Autodesk Inventor part; units mm, degrees
ref_plane "YZ Plane" through (0, 0, 0) normal (1, 0, 0) x (0, 1, 0)
ref_plane "XZ Plane" through (0, 0, 0) normal (0, 1, 0) x (-1, 0, 0)
ref_plane "XY Plane" through (0, 0, 0) normal (0, 0, 1) x (1, 0, 0)
sketch "Sketch1" plane through (0, 0, 0) normal (0, 0, 1) x (1, 0, 0)
  line L0 (0, 0) -> (76.2, 0)
  line L1 (0, 0) -> (0, -50.8)
  line L2 (0, -50.8) -> (12.7, -50.8)
  line L3 (18.3796, -49.4592) -> (69.1796, -24.0592)
  arc A0 (12.7, -50.8) -> (18.3796, -49.4592) centre (12.7, -38.1) ccw
  line L4 (76.2, 0) -> (76.2, -12.7)
  arc A1 (69.1796, -24.0592) -> (76.2, -12.7) centre (63.5, -12.7) ccw
  circle A2 centre (12.7, -38.1) radius 4.8006
  circle A3 centre (12.7, -12.7) radius 4.8006
  circle A4 centre (63.5, -12.7) radius 4.8006
  line L5 (12.7, -12.7) -> (63.5, -12.7) construction
  line L6 (12.7, -38.1) -> (12.7, -12.7) construction
  circle A5 centre (38.1, -25.4) radius 3.175
  dimension "d2" = 50.8
  dimension "d3" = 12.7
  dimension "d4" = 12.7
  dimension "d5" = 12.7
  dimension "d7" = 9.6012
  dimension "d8" = 25.4
  dimension "d10" = 50.8
  dimension "d11" = 12.7
  dimension "d12" = 6.35
  dimension "d13" = 12.7
  dimension "d14" = 25.4
  dimension "d15" = 12.7
  dimension "d16" = 76.2
extrude "Extrusion1" add sketch "Sketch1" along normal mid plane 9.525
properties part number "Plate"
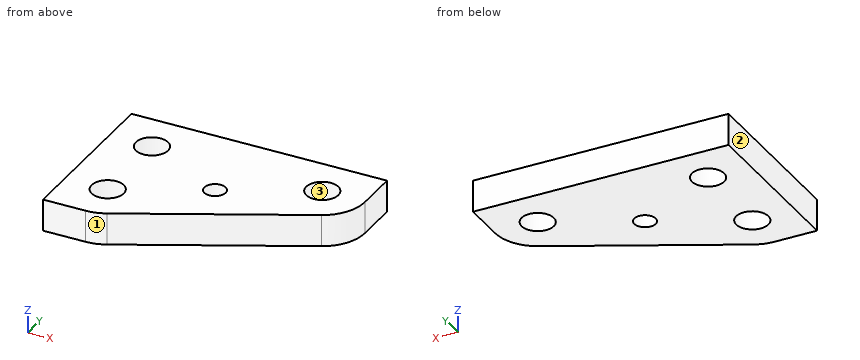
Verification items for the finished model (mm, model axes). Face numbers are marked on the shaded views. Round coordinates to 2 decimals unless told otherwise and drop trailing zeros. Loops run counter-clockwise (first coordinate to the right, second up) from the corner with the lowest first, then second, coordinate; pieces in that order, holes last. Notation, with made-up numbers: (64, 79.25) - (71, 79.25) arc R28 ccw to (71, 115.25) - close; hole circle Ø8 at (68.25, 61.5). An arc over 180 degrees is marked (long way). Answer in a Markdown table with one row per item. Add a question column.
Q1. Section check D-D on x = 15. Enter the section's corners in (y, z), plus the area to 3 significant figures.
Q2. Material ranges on line 1 (Y direction, x = 12.7, z = -2.5); line 2 (X direction, y = -17, z = 1.5); line 3 (X direction, y = -12, z = 4), recorded low to high.
Q3. Section check B-B on x = 60. Enter the section's corners in (y, z), plus the area to 3 significant figures.
Q4. Section check C-C on y = -38.1. Enter the section's corners in (x, z), plus the area to 3 significant figures.
Q5. Release check for a two-part mould opening along X. For the marked faces 1, 2 and 3 record: pulls with the +X half, pulls with the -X half, needs draft (parallel to the pull), parting line crosses it, or undercut.
Q6. Section check A-A on z = -2.25. Enter the section's corners in (x, y) (3 decimals).
Q7. Gauge pin test, flat end, axial feed: pin 1 (4 mm diameter, centred on y = -32.5, z = 3, fed in from -X). Record the tip position at first contact, or that the pin passes through.
Found:
| question | item | result |
|---|---|---|
| 1 | outline | (-50.59, -4.76) - (-42.31, -4.76) - (-42.31, 4.76) - (-50.59, 4.76) - close; (-33.89, -4.76) - (-16.91, -4.76) - (-16.91, 4.76) - (-33.89, 4.76) - close; (-8.49, -4.76) - (0, -4.76) - (0, 4.76) - (-8.49, 4.76) - close |
| 1 | area | 321 mm² |
| 2 | line 1 | y = -50.8 to -42.9, -33.3 to -17.5, -7.9 to 0 |
| 2 | line 2 | x = 0 to 10.57, 14.83 to 61.37, 65.63 to 75.45 |
| 2 | line 3 | x = 0 to 7.95, 17.45 to 58.75, 68.25 to 76.2 |
| 3 | outline | (-28.65, -4.76) - (-15.99, -4.76) - (-15.99, 4.76) - (-28.65, 4.76) - close; (-9.41, -4.76) - (0, -4.76) - (0, 4.76) - (-9.41, 4.76) - close |
| 3 | area | 210 mm² |
| 4 | outline | (0, -4.76) - (7.9, -4.76) - (7.9, 4.76) - (0, 4.76) - close; (17.5, -4.76) - (41.1, -4.76) - (41.1, 4.76) - (17.5, 4.76) - close |
| 4 | area | 300 mm² |
| 5 | face 1 | pulls with the +X half |
| 5 | face 2 | pulls with the -X half |
| 5 | face 3 | undercut |
| 6 | outline | (0, -50.8) - (12.7, -50.8) arc R12.699 ccw to (18.38, -49.459) - (69.18, -24.059) arc R12.7 ccw to (76.2, -12.7) - (76.2, 0) - (0, 0) - close; hole circle Ø9.601 at (12.7, -38.1); hole circle Ø9.601 at (12.7, -12.7); hole circle Ø6.35 at (38.1, -25.4); hole circle Ø9.601 at (63.5, -12.7) |
| 7 | pin 1 | stops at x = 0 |
